The drawing under review shows one solid part. Ordinate dimensions are in mm from its lowest x, y, z. Coordinates: 2 decimals unless noted, no trailing zeros. Order: outer loops, then holes, each group sorted by start corner. A loop starts at its lowest first (then second) coordinate and runs counter-clockwise, first axis right, second up.
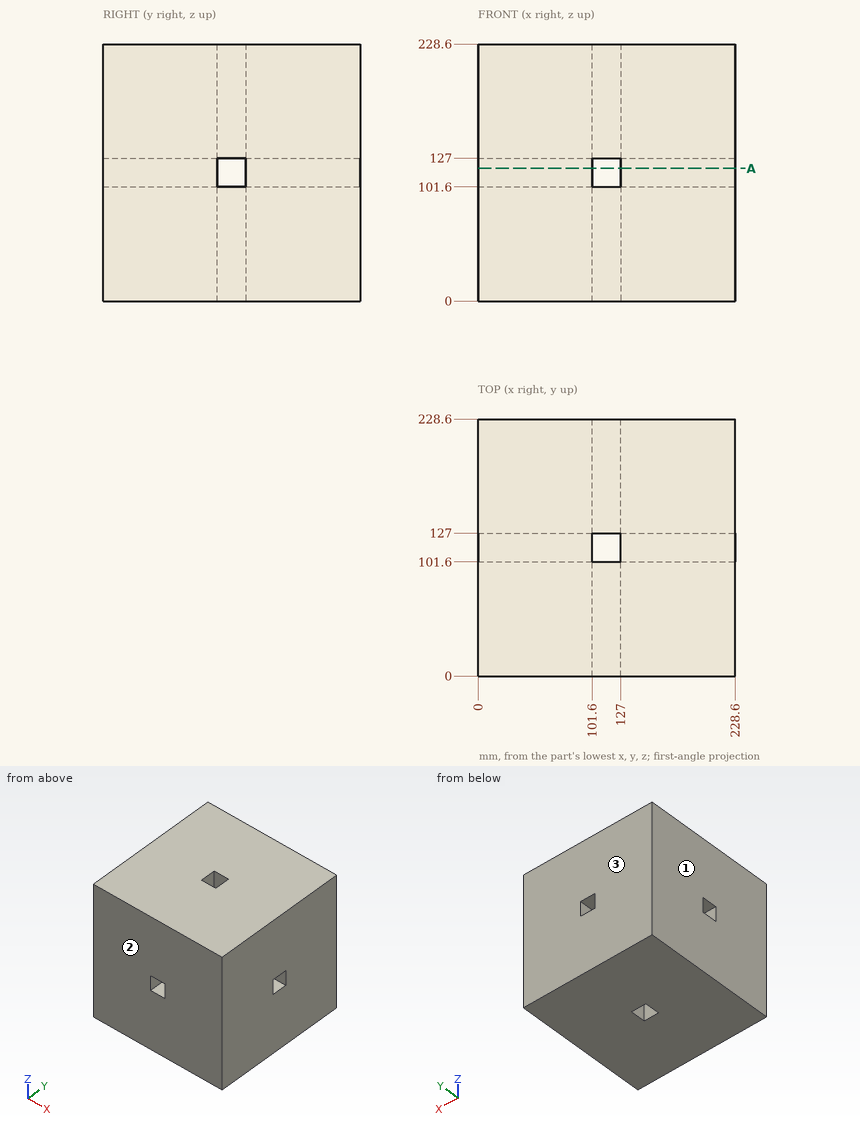
(1) Wall thickness on line 1 (X direction, y = 108.5, z = 90.5): over which ranges is the line inside the solid? List them lowest first.
(2) The part is to be moulded in two halves that separate along Y. For the marked faces 1, 2 and 3, say which applies: +Y half, -Y half, draft (parallel to the pull), parting line (faces both ways), or undercut.
(3) Consider section A-A (z = 118). Give the boundary of the cut face in (x, y), then the cut area to 3 significant figures.
Findings:
1. line 1: x = 0 to 101.6, 127 to 228.6
2. face 1: draft
2. face 2: -Y half
2. face 3: +Y half
3. outline: (0, 0) - (101.6, 0) - (101.6, 101.6) - (0, 101.6) - close; (0, 127) - (101.6, 127) - (101.6, 228.6) - (0, 228.6) - close; (127, 0) - (228.6, 0) - (228.6, 101.6) - (127, 101.6) - close; (127, 127) - (228.6, 127) - (228.6, 228.6) - (127, 228.6) - close
3. area: 41,300 mm2
